The listing builds one solid part. Answer for the finished solid, in the listing's coordinates (mm). A direction names the side the tool comes from. Give positions to 0.01 mm unless a question says otherwise; leave off trailing zeros. Write each loop counter-clockwise with the first axis right and the second up, starting at its lowest first coordinate (ties: lowest second). Pieces come first, ordered by that corner, then holes. Notation, with made-up numbers: (13.25, 37.25) -> (59.25, 37.25) arc R25 ccw to (59.25, 66.25) -> close; hole circle Ø8 at (-36.75, 77). An arc over 180 degrees is marked (long way). Put each result on its own line as item: value. Start each with the question number.
1) A cutting plane is placed at A-A (y = -9.5). Write down the section's boundary in (x, z).
2) For faces 1 (the flat face through (53.52, -9, 2)), 2 (the flat face through (18, -32, 0)), determine the directions among +Z, -Z, +X, -X, +Y, -Y from which every point of the face is accessible in a straight line to the end or side of a thin tool.
3) A cutting plane is placed at B-B (x = 56.07). Write down the section's boundary in (y, z).
4) A cutting plane is placed at D-D (y = -47.5). Write down the section's boundary in (x, z), then the cut area to 3 significant figures.
5) Find the intervals of material crossed by line 1 along X through (y, z) = (-57, 3.55); line 2 along X through (y, z) = (-34.5, 2.6); line 3 along Y through (x, z) = (7, 1.4), in increasing order. Write a range as from..to.
6) For a pull along Y with two mould halves and no side action, classify faces 3 (the flat face through (44, -32, 3)), 4 (the flat face through (65, -33, 2)) as released by +Y, released by -Y, zero draft, split by the parting line, or undercut.
7) A cutting plane is placed at C-C (z = 2.2). Write down the section's boundary in (x, y), then the cut area to 3 significant figures.
from build123d import *

# Parameters (mm, degrees)
SKETCH1_W           = 65
SKETCH1_H           = 65
BOSS_EXTRUDE1_DEPTH = 5
CUT_EXTRUDE2_REACH  = 94.06


with BuildPart() as part:
    # Sketch1 → Boss-Extrude1 (new body)
    with BuildSketch(Plane.XY):
        with Locations((32.5, -32.5)):
            Rectangle(SKETCH1_W, SKETCH1_H)
        with BuildLine():
            Line((11.48, -3.93), (11.48, -13.93))
            ThreePointArc((11.48, -13.93), (8.93, -16.48), (6.38, -13.93))
            Line((6.38, -13.93), (6.38, -3.93))
            ThreePointArc((6.38, -3.93), (8.93, -1.38), (11.48, -3.93))
        make_face(mode=Mode.SUBTRACT)
        with BuildLine():
            Line((53.52, -3.93), (53.52, -13.93))
            ThreePointArc((53.52, -13.93), (56.07, -16.48), (58.62, -13.93))
            Line((58.62, -13.93), (58.62, -3.93))
            ThreePointArc((58.62, -3.93), (56.07, -1.38), (53.52, -3.93))
        make_face(mode=Mode.SUBTRACT)
        with BuildLine():
            Line((11.48, -61.07), (11.48, -51.07))
            ThreePointArc((11.48, -51.07), (8.93, -48.52), (6.38, -51.07))
            Line((6.38, -51.07), (6.38, -61.07))
            ThreePointArc((6.38, -61.07), (8.93, -63.62), (11.48, -61.07))
        make_face(mode=Mode.SUBTRACT)
        with BuildLine():
            Line((53.52, -61.07), (53.52, -51.07))
            ThreePointArc((53.52, -51.07), (56.07, -48.52), (58.62, -51.07))
            Line((58.62, -51.07), (58.62, -61.07))
            ThreePointArc((58.62, -61.07), (56.07, -63.62), (53.52, -61.07))
        make_face(mode=Mode.SUBTRACT)
    extrude(amount=BOSS_EXTRUDE1_DEPTH)

    # Sketch2 → Cut-Extrude2 (cut, up to next)
    with BuildSketch(Plane.XY.offset(5), mode=Mode.PRIVATE) as cut_extrude2_sk1:
        with BuildLine():
            Line((44, -27.5), (44, -37.5))
            ThreePointArc((44, -37.5), (32.5, -49), (21, -37.5))
            Line((21, -37.5), (21, -27.5))
            ThreePointArc((21, -27.5), (32.5, -16), (44, -27.5))
        make_face()
    cut_extrude2_tool1 = extrude(cut_extrude2_sk1.sketch, amount=-CUT_EXTRUDE2_REACH, mode=Mode.PRIVATE) & part.part
    add(cut_extrude2_tool1.solids().sort_by_distance((32.5, -32.5, 5))[0], mode=Mode.SUBTRACT)


solid = part.part
Reply:
1. outline: (0, 0) -> (6.38, 0) -> (6.38, 5) -> (0, 5) -> close; (11.48, 0) -> (53.52, 0) -> (53.52, 5) -> (11.48, 5) -> close; (58.62, 0) -> (65, 0) -> (65, 5) -> (58.62, 5) -> close
2. face 1: +Z, -Z
2. face 2: -Z, +X, -X, +Y, -Y
3. outline: (-65, 0) -> (-63.62, 0) -> (-63.62, 5) -> (-65, 5) -> close; (-48.52, 0) -> (-16.48, 0) -> (-16.48, 5) -> (-48.52, 5) -> close; (-1.38, 0) -> (0, 0) -> (0, 5) -> (-1.38, 5) -> close
4. outline: (0, 0) -> (26.82, 0) -> (26.82, 5) -> (0, 5) -> close; (38.18, 0) -> (65, 0) -> (65, 5) -> (38.18, 5) -> close
4. area: 268 mm2
5. line 1: x = 0..6.38, 11.48..53.52, 58.62..65
5. line 2: x = 0..21, 44..65
5. line 3: y = -65..-62.74, -49.4..-15.6, -2.26..0
6. face 3: undercut
6. face 4: zero draft
7. outline: (0, -65) -> (65, -65) -> (65, 0) -> (0, 0) -> close; hole (6.38, -61.07) arc R2.55 ccw to (11.48, -61.07) -> (11.48, -51.07) arc R2.55 ccw to (6.38, -51.07) -> close; hole (6.38, -13.93) arc R2.55 ccw to (11.48, -13.93) -> (11.48, -3.93) arc R2.55 ccw to (6.38, -3.93) -> close; hole (21, -37.5) arc R11.5 ccw to (44, -37.5) -> (44, -27.5) arc R11.5 ccw to (21, -27.5) -> close; hole (53.52, -61.07) arc R2.55 ccw to (58.62, -61.07) -> (58.62, -51.07) arc R2.55 ccw to (53.52, -51.07) -> close; hole (53.52, -13.93) arc R2.55 ccw to (58.62, -13.93) -> (58.62, -3.93) arc R2.55 ccw to (53.52, -3.93) -> close
7. area: 3,290 mm2
